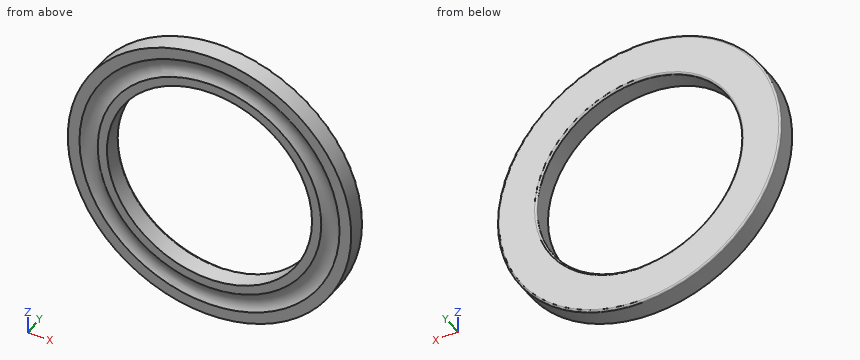
```python
from build123d import *

# Parameters (mm, degrees)
SKETCH1_R           = 85
SKETCH1_R_2         = 61.5
BOSS_EXTRUDE1_DEPTH = 12.2
FILLET1_R           = 1.1


with BuildPart() as part:
    # Sketch1 → Boss-Extrude1 (new body)
    with BuildSketch(Plane(origin=(0, 0, 0), x_dir=(1, 0, 0), z_dir=(0, 1, 0))):
        Circle(SKETCH1_R)
        Circle(SKETCH1_R_2, mode=Mode.SUBTRACT)
    extrude(amount=BOSS_EXTRUDE1_DEPTH)

    # Fillet1
    fillet1_edges = [part.edges().sort_by_distance(p)[0] for p in [
        (-85, 12.2, 0),
        (-61.5, 12.2, 0),
    ]]
    fillet(fillet1_edges, radius=FILLET1_R)

    # Sketch2 → Cut-Revolve1 (revolve, cut)
    with BuildSketch(Plane.XY):
        with BuildLine():
            Line((-77.98, 0), (-67.02, 0))
            ThreePointArc((-67.02, 0), (-72.5, 1.827500428), (-77.98, 0))
        make_face()
    revolve(axis=Axis((0, 11.1, 0), (0, -1, 0)), mode=Mode.SUBTRACT)


solid = part.part
```
Build history of the part. All positions in model axes, mm. Give positions to 0.01 mm unless a question says otherwise; leave off trailing zeros. Loops run counter-clockwise (first coordinate to the right, second up) from the corner with the lowest first, then second, coordinate; pieces in that order, holes last. Notation, with made-up numbers: (85.5, 35.25) - (126.5, 35.25) arc R14 ccw to (126.5, 51.25) - close; hole circle Ø4 at (-11.5, -27). An arc over 180 degrees is marked (long way). Use a Markdown table: item, result.
(1) Band-saw the part on A-A (z = 0). Give the cut face in (x, y).
Taken from the geometry:
| item | result |
|---|---|
| outline | (-85, 0) - (-77.98, 0) arc R9.13 cw to (-67.02, 0) - (-61.5, 0) - (-61.5, 11.1) arc R1.1 ccw to (-62.6, 12.2) - (-83.9, 12.2) arc R1.1 ccw to (-85, 11.1) - close; (61.5, 0) - (67.02, 0) arc R9.13 cw to (77.98, 0) - (85, 0) - (85, 11.1) arc R1.1 ccw to (83.9, 12.2) - (62.6, 12.2) arc R1.1 ccw to (61.5, 11.1) - close |
(2) Band-saw the part on C-C (y = 8.5). Give the cut face in (x, z).
Taken from the geometry:
| item | result |
|---|---|
| outline | circle Ø170 at (0, 0); hole circle Ø123 at (0, 0) |
(3) Band-saw the part on B-B (x = 0). Give the cut face in (y, z), and give its area (3 significant figures).
Taken from the geometry:
| item | result |
|---|---|
| outline | (0, -85) - (11.1, -85) arc R1.1 ccw to (12.2, -83.9) - (12.2, -62.6) arc R1.1 ccw to (11.1, -61.5) - (0, -61.5) - (0, -67.02) arc R9.13 cw to (0, -77.98) - close; (0, 61.5) - (11.1, 61.5) arc R1.1 ccw to (12.2, 62.6) - (12.2, 83.9) arc R1.1 ccw to (11.1, 85) - (0, 85) - (0, 77.98) arc R9.13 cw to (0, 67.02) - close |
| area | 545 mm2 |
(4) Drop flat-ended pins along their axis: pin 1 Ø2 at (x, y) = (-16.5, 3.5) entering from +Z; pin 2 Ø6 at (x, y) = (63, 8.5) entering from -Z; pin 3 Ø1.5 at (x, y) = (-58, 4.5) entering from +Z. Give the stop position or say it passes through.
Taken from the geometry:
| item | result |
|---|---|
| pin 1 | z = 83.57 |
| pin 2 | z = -60.21 |
| pin 3 | z = 62.83 |
(5) Wall check: line 1 along X through (y, z) = (6.25, 0); line 2 along Z through (x, y) = (-37.5, 7.5). Give the ranges that are in metal, low to high.
Taken from the geometry:
| item | result |
|---|---|
| line 1 | -85 to -61.5, 61.5 to 85 |
| line 2 | -76.28 to -48.74, 48.74 to 76.28 |
